```python
from build123d import *

# Parameters (mm, degrees)
SKETCH_2_W               = 11
SKETCH_2_H               = 18
EXTRUDE_1_DEPTH          = 0.8
SKETCH_3_W               = 10
SKETCH_3_H               = 11
EXTRUDE_3_DEPTH          = 2.3
SKETCH_7_R               = 0.35
CUT_EXTRUDE_1_DEPTH      = 2.3
SKETCH_9_R               = 0.35
CUT_EXTRUDE_2_DEPTH      = 2.3
CUT_EXTRUDE_2_DEPTH_BACK = 2.3
SKETCH_10_R              = 0.35
CUT_EXTRUDE_5_DEPTH      = 2.3
CUT_EXTRUDE_5_DEPTH_BACK = 2.3


with BuildPart() as part:
    # 草图2 → 凸台-拉伸1 (new body)
    with BuildSketch(Plane(origin=(0, 0, 0), x_dir=(1, 0, 0), z_dir=(0, 1, 0))):
        Rectangle(SKETCH_2_W, SKETCH_2_H)
    extrude(amount=EXTRUDE_1_DEPTH)

    # 草图3 → 凸台-拉伸3 (add)
    with BuildSketch(Plane(origin=(0, 0, 0), x_dir=(1, 0, 0), z_dir=(0, 1, 0))):
        with Locations((0, 2.5)):
            Rectangle(SKETCH_3_W, SKETCH_3_H)
    extrude(amount=EXTRUDE_3_DEPTH)

    # 草图7 → 切除-拉伸1 (cut)
    with BuildSketch(Plane(origin=(0, 0.8, 0), x_dir=(1, 0, 0), z_dir=(0, 1, 0))):
        with Locations((-3.75, 9)):
            Circle(SKETCH_7_R)
    extrude(amount=-CUT_EXTRUDE_1_DEPTH, mode=Mode.SUBTRACT)

    # 草图9 → 切除-拉伸2 (cut, two sides)
    with BuildSketch(Plane(origin=(0, 0, 0), x_dir=(1, 0, 0), z_dir=(0, 1, 0))) as cut_extrude_2_sk:
        with Locations((-2.25, 9)):
            Circle(SKETCH_9_R)
        with Locations((-0.75, 9)):
            Circle(SKETCH_9_R)
        with Locations((0.75, 9)):
            Circle(SKETCH_9_R)
        with Locations((3.75, 9)):
            Circle(SKETCH_9_R)
        with Locations((2.25, 9)):
            Circle(SKETCH_9_R)
    extrude(amount=CUT_EXTRUDE_2_DEPTH, mode=Mode.SUBTRACT)
    extrude(cut_extrude_2_sk.sketch, amount=-CUT_EXTRUDE_2_DEPTH_BACK, mode=Mode.SUBTRACT)

    # 草图10 → 切除-拉伸5 (cut, two sides)
    with BuildSketch(Plane(origin=(0, 0, 0), x_dir=(1, 0, 0), z_dir=(0, 1, 0))) as cut_extrude_5_sk:
        with Locations((-5.5, 7.25)):
            Circle(SKETCH_10_R)
        with Locations((5.5, 7.25)):
            Circle(SKETCH_10_R)
        with Locations((5.5, -0.25)):
            Circle(SKETCH_10_R)
        with Locations((-5.5, 2.75)):
            Circle(SKETCH_10_R)
        with Locations((5.5, 5.75)):
            Circle(SKETCH_10_R)
        with Locations((-5.5, 4.25)):
            Circle(SKETCH_10_R)
        with Locations((5.5, 2.75)):
            Circle(SKETCH_10_R)
        with Locations((-5.5, 5.75)):
            Circle(SKETCH_10_R)
        with Locations((5.5, 4.25)):
            Circle(SKETCH_10_R)
        with Locations((5.5, 1.25)):
            Circle(SKETCH_10_R)
        with Locations((-5.5, 1.25)):
            Circle(SKETCH_10_R)
        with Locations((-5.5, -0.25)):
            Circle(SKETCH_10_R)
    extrude(amount=CUT_EXTRUDE_5_DEPTH, mode=Mode.SUBTRACT)
    extrude(cut_extrude_5_sk.sketch, amount=-CUT_EXTRUDE_5_DEPTH_BACK, mode=Mode.SUBTRACT)


solid = part.part
```
Can you work these out from the model? Positions are in its coordinate system, mm. A direction names the side the tool comes from. Give positions to 0.01 mm unless a question says otherwise; leave off trailing zeros. Loops run counter-clockwise (first coordinate to the right, second up) from the corner with the lowest first, then second, coordinate; pieces in that order, holes last. Notation, with made-up numbers: M -38.5,-8.5 L -26.5,-8.5 A14 ccw -26.5,-0.5 Z; hole C 8.5,-40 d2. An arc over 180 degrees is marked long. Use one line per item in the form item = value. Start each with the question number.
(1) On a 3-axis mill with a long thin cutter (end or side, diameter ignored), from which of +Z, -Z, +X, -X, +Y, -Y can I reach the whole of each face in a straight line? I mean faces 1 (the flat face through (5, 2, -2)), 2 (the flat face through (0, 2, -8)), 3 (the flat face through (0, 2.3, -3)), 4 (the flat face through (-5, 2, -2)), 5 (the flat face through (0, 2, 3)). Say none if no direction works.
(2) I'm going to push a flat-ended pin straight in: P1, Ø1.2, axis at x = 0, y = 1.5, coming from the +Z side. Where does the tip first touch, or does it pass through?
(3) Please list where these lines run through material, in increasing order: line 1 (Z direction, x = 4, y = 0.95); line 2 (X direction, y = 0.25, z = -4.25); line 3 (Y direction, x = 1, z = 7.25).
(4) I want a section at C-C, the plane y = 1.65. Write out the boundary of the cut face in (x, z), and give its area (3 significant figures).
(5) I want a section at D-D, the plane z = 7.25. Write out the boundary of the cut face in (x, y), and give its area (3 significant figures).
(6) I want a section at B-B, the plane z = 0.25. Write out the boundary of the cut face in (x, y).
(7) I want a section at A-A, the plane x = -3. Write out the boundary of the cut face in (y, z).
Worked out:
q1.face_1 = +Z, -Z, +X, +Y
q1.face_2 = -Z, +X, -X, +Y
q1.face_3 = +Z, -Z, +X, -X, +Y
q1.face_4 = +Z, -Z, -X, +Y
q1.face_5 = +Z, +X, -X, +Y
q2.P1 = 3
q3.line_1 = -8 to 3
q3.line_2 = -5.15 to 5.15
q3.line_3 = 0 to 0.8
q4.outline = M -5,-8 L 5,-8 L 5,3 L -5,3 Z
q4.area = 110 mm²
q5.outline = M -5.5,0 L 5.5,0 L 5.5,0.8 L -5.5,0.8 Z
q5.area = 8.80 mm²
q6.outline = M -5.15,0 L 5.15,0 L 5.15,0.8 L 5,0.8 L 5,2.3 L -5,2.3 L -5,0.8 L -5.15,0.8 Z
q7.outline = M 0,-9 L 0.8,-9 L 0.8,-8 L 2.3,-8 L 2.3,3 L 0.8,3 L 0.8,9 L 0,9 Z
